Solid Edge part; units mm, degrees
sketch "Sketch1" plane through (0, 0, 0) normal (0, 0, 1) x (1, 0, 0)
  line L0 (8.5, 7.5) -> (8.5, -7.5)
  line L1 (8.5, -7.5) -> (11, -7.5)
  line L2 (11, -11) -> (11, -7.5)
  line L3 (-11, -11) -> (11, -11)
  line L4 (-11, 11) -> (-11, -11)
  line L5 (11, 11) -> (-11, 11)
  line L6 (11, 7.5) -> (11, 11)
  line L7 (11, 7.5) -> (8.5, 7.5)
  line L8 (17.5, -17.5) -> (17.5, 17.5)
  line L9 (17.5, 17.5) -> (-17.5, 17.5)
  line L10 (-17.5, 17.5) -> (-17.5, -17.5)
  line L11 (-17.5, -17.5) -> (17.5, -17.5)
extrude "Protrusion1" add sketch "Sketch1" along normal blind 10
chamfer "Chaflán_1" distance 2 angle 45 12 edges at (17.5, -17.5, 5) (-17.5, -17.5, 5) (-17.5, 17.5, 5) (17.5, 17.5, 5) (0, 17.5, 10) (-17.5, 0, 10) (0, 17.5, 0) (-17.5, 0, 0) (0, -17.5, 0) (17.5, 0, 0) (17.5, 0, 10) (0, -17.5, 10)
sketch "Sketch2" plane through (17.5, 0, 5) normal (1, 0, 0) x (0, 1, 0)
  circle A0 centre (0, 0) radius 2.25
extrude "Cutout1" cut sketch "Sketch2" against normal up to surface (9 mm away)
The model under review builds one solid part; all positions refer to its coordinate system, in mm. A direction names the side the tool comes from. Give positions to 0.01 mm unless a question says otherwise; leave off trailing zeros. Write each loop counter-clockwise with the first axis right and the second up, starting at its lowest first coordinate (ties: lowest second). Pieces come first, ordered by that corner, then holes. Notation, with made-up numbers: M 36,51.25 L 65,51.25 A32 cw 65,90.25 Z; hole C 86,-20 d11. An arc over 180 degrees is marked long. Answer in a Markdown table with one row per item.
Item 1: Add section C-C on y = 0. Give the boundary of the cut face in (x, z), plus the area to 4 significant figures.
Check sheet entries:
| item | result |
|---|---|
| outline | M -17.5,2 L -15.5,0 L -11,0 L -11,10 L -15.5,10 L -17.5,8 Z; M 8.5,0 L 15.5,0 L 17.5,2 L 17.5,2.75 L 8.5,2.75 Z; M 8.5,7.25 L 17.5,7.25 L 17.5,8 L 15.5,10 L 8.5,10 Z |
| area | 106.5 mm2 |
Item 2: Draft analysis for pull direction Z (two halves, no side actions). For faces 1 (the face through (13.06, -0.29, 7.23)), 2 (the face through (0, -11, 5)), 3 (the face through (0.2, 16.5, 1)), state which applies: +Z half, -Z half, draft (parallel to the pull), parting line (faces both ways), or undercut.
Check sheet entries:
| item | result |
|---|---|
| face 1 | undercut |
| face 2 | draft |
| face 3 | -Z half |
Item 3: Add section D-D on x = 11.5. Give the boundary of the cut face in (y, z), plus the area to 3 significant figures.
Check sheet entries:
| item | result |
|---|---|
| outline | M -17.5,2 L -15.5,0 L 15.5,0 L 17.5,2 L 17.5,8 L 15.5,10 L -15.5,10 L -17.5,8 Z; hole C 0,5 d4.5 |
| area | 326 mm2 |
Item 4: Tool access review of faces 4 (the face through (8.5, 2, 3)), 5 (the face through (16.5, -0.2, 9)): name each direction out of +Z, -Z, +X, -X, +Y, -Y from which nothing blocks a thin tool from reaching the whole face with its end or side.
Check sheet entries:
| item | result |
|---|---|
| face 4 | +Z, -Z |
| face 5 | +Z, +X, +Y, -Y |
Item 5: Add section A-A on y = 10.5. Give the boundary of the cut face in (x, z), plus the area to 3 significant figures.
Check sheet entries:
| item | result |
|---|---|
| outline | M -17.5,2 L -15.5,0 L -11,0 L -11,10 L -15.5,10 L -17.5,8 Z; M 11,0 L 15.5,0 L 17.5,2 L 17.5,8 L 15.5,10 L 11,10 Z |
| area | 122 mm2 |
Item 6: For line 1 along Z through (x, y) = (13, 0); line 2 along Y through (x, z) = (-2.5, 2.75), list the stretches that pass through material, from the lowest coordinate up.
Check sheet entries:
| item | result |
|---|---|
| line 1 | 0 to 2.75, 7.25 to 10 |
| line 2 | -17.5 to -11, 11 to 17.5 |
